Build history of the part. All positions in model axes, mm. Face numbers are marked on the shaded views. A direction names the side the tool comes from. Round coordinates to 2 decimals unless told otherwise and drop trailing zeros. Write each loop counter-clockwise with the first axis right and the second up, starting at its lowest first coordinate (ties: lowest second). Pieces come first, ordered by that corner, then holes. Notation, with made-up numbers: M 47.25,-29 L 71.25,-29 A23 ccw 71.25,2 Z; hole C 51.5,44 d1. An arc over 180 degrees is marked long. One line per item, written item: value. Start each with the question number.
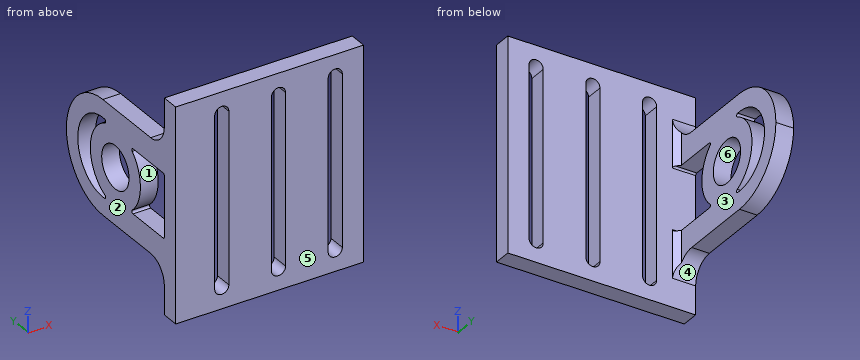
```python
from build123d import *

# Parameters (mm, degrees)
SKETCH1_W           = 48
SKETCH1_H           = 60
BOSS_EXTRUDE1_DEPTH = 5
SKETCH2_W           = 60
SKETCH2_H           = 5
BOSS_EXTRUDE2_DEPTH = 5
SKETCH4_W           = 5
SKETCH4_H           = 32
BOSS_EXTRUDE3_DEPTH = 43
FILLET2_R           = 6
CHAMFER1_SIZE       = 1.5
SKETCH6_R           = 6
CUT_EXTRUDE1_DEPTH  = 94.343451832
FILLET3_R           = 16
CUT_EXTRUDE2_DEPTH  = 94.343451832


with BuildPart() as part:
    # Sketch1 → Boss-Extrude1 (new body)
    with BuildSketch(Plane(origin=(0, 0, 0), x_dir=(1, 0, 0), z_dir=(0, 1, 0))):
        with Locations((24, -30)):
            Rectangle(SKETCH1_W, SKETCH1_H)
        with BuildLine():
            Line((10, -6), (10, -54))
            ThreePointArc((10, -54), (8, -56), (6, -54))
            Line((6, -54), (6, -6))
            ThreePointArc((6, -6), (8, -4), (10, -6))
        make_face(mode=Mode.SUBTRACT)
        with BuildLine():
            Line((38, -6), (38, -54))
            ThreePointArc((38, -54), (40, -56), (42, -54))
            Line((42, -54), (42, -6))
            ThreePointArc((42, -6), (40, -4), (38, -6))
        make_face(mode=Mode.SUBTRACT)
        with BuildLine():
            Line((26, -6), (26, -54))
            ThreePointArc((26, -54), (24, -56), (22, -54))
            Line((22, -54), (22, -6))
            ThreePointArc((22, -6), (24, -4), (26, -6))
        make_face(mode=Mode.SUBTRACT)
    extrude(amount=BOSS_EXTRUDE1_DEPTH)

    # Sketch2 → Boss-Extrude2 (add)
    with BuildSketch(Plane.ZY):
        with Locations((30, 2.5)):
            Rectangle(SKETCH2_W, SKETCH2_H)
    extrude(amount=BOSS_EXTRUDE2_DEPTH)

    # Sketch4 → Boss-Extrude3 (add)
    with BuildSketch(Plane(origin=(0, 5, 0), x_dir=(1, 0, 0), z_dir=(0, 1, 0))):
        with Locations((-2.5, -30)):
            Rectangle(SKETCH4_W, SKETCH4_H)
    extrude(amount=BOSS_EXTRUDE3_DEPTH)

    # Fillet2
    fillet2_edges = [part.edges().sort_by_distance(p)[0] for p in [
        (-2.5, 5, 46),
        (-2.5, 5, 14),
    ]]
    fillet(fillet2_edges, radius=FILLET2_R)

    # Chamfer1
    chamfer1_edges = [part.edges().sort_by_distance(p)[0] for p in [
        (0, 5, 30),
    ]]
    chamfer(chamfer1_edges, length=CHAMFER1_SIZE)

    # Sketch6 → Cut-Extrude1 (cut, through all)
    with BuildSketch(Plane.ZY.offset(5)):
        with Locations((30, 26.5)):
            Circle(SKETCH6_R)
    extrude(amount=-CUT_EXTRUDE1_DEPTH, mode=Mode.SUBTRACT)

    # Fillet3
    fillet3_edges = [part.edges().sort_by_distance(p)[0] for p in [
        (-2.5, 48, 46),
        (-2.5, 48, 14),
    ]]
    fillet(fillet3_edges, radius=FILLET3_R - 0.0001)  # a hair under: the kernel refuses the full size

    # Sketch7 → Cut-Extrude2 (cut, through all)
    with BuildSketch(Plane.ZY.offset(5)):
        with BuildLine():
            Line((21, 18.754033308), (21, 5.5))
            ThreePointArc((21, 5.5), (21.146446609, 5.146446609), (21.5, 5))
            Line((21.5, 5), (38.5, 5))
            ThreePointArc((38.5, 5), (38.853553391, 5.146446609), (39, 5.5))
            Line((39, 5.5), (39, 18.754033308))
            ThreePointArc((39, 18.754033308), (38.68057878, 19.220285712), (38.130434783, 19.090814468))
            ThreePointArc((38.130434783, 19.090814468), (30, 15.5), (21.869565217, 19.090814468))
            ThreePointArc((21.869565217, 19.090814468), (21.31942122, 19.220285712), (21, 18.754033308))
        make_face()
        with BuildLine():
            ThreePointArc((40.971902892, 31.214285714), (30, 43), (19.028097108, 31.214285714))
            ThreePointArc((19.028097108, 31.214285714), (19.438706545, 30.757825209), (19.982175621, 31.043478261))
            ThreePointArc((19.982175621, 31.043478261), (30, 37.5), (40.017824379, 31.043478261))
            ThreePointArc((40.017824379, 31.043478261), (40.561293455, 30.757825209), (40.971902892, 31.214285714))
        make_face()
    extrude(amount=-CUT_EXTRUDE2_DEPTH, mode=Mode.SUBTRACT)


solid = part.part
```
Item 1: Cut at A-A, the plane y = 26.5. Write the cut outline in (x, z).
Item 2: Which spindle directions (+Z, -Z, +X, -X, +Y, -Y) get a long thin tool onto all of the face, cutting with end or side? Do the marked faces 1 and 2. Say none if no direction does.
Item 3: Two-plate mould, pull along Y, no slides. Class the marked faces 3, 4, 5 and 6: pulls with the +Y half, pulls with the -Y half, needs draft (parallel to the pull), parting line crosses it, or undercut.
Item 4: Drop flat-ended pins along their axis: pin 1 (4 mm diameter, centred on x = -2.5, y = 23.5, fed in from +Z); pin 2 (2 mm diameter, centred on y = 32, z = 24.5, fed in from +X); pin 3 (3 mm diameter, centred on x = -0.5, y = 10.5, fed in from -Z); pin 4 (7 mm diameter, centred on y = 26.5, z = 30, fed in from +X). Give the stop position or say it passes through.
Item 5: Cut at D-D, the plane y = 44.5. Write the cut outline in (x, z).
Item 6: Cut at B-B, the plane x = 40. Write the cut outline in (y, z).
Item 7: Drill centre lines: line 1 (Y direction, x = 12, z = 28); line 2 (X direction, y = 39.5, z = 42.5); line 3 (Z direction, x = -1, y = 26). Where is each one in solid material? Low to high.
Item 8: Cut at C-C, the plane x = 31. Write the cut outline in (y, z), plus the area to 3 significant figures.
Computed values:
1. outline: M -5,14 L 0,14 L 0,24 L -5,24 Z; M -5,36 L 0,36 L 0,46 L -5,46 Z
2. face 1: +X, -X
2. face 2: +Z, -Z, -X, +Y, -Y
3. face 3: needs draft
3. face 4: pulls with the +Y half
3. face 5: pulls with the -Y half
3. face 6: undercut
4. pin 1: stops at z = 46
4. pin 2: stops at x = 0
4. pin 3: stops at z = 13.66
4. pin 4: passes through
5. outline: M -5,20.01 L 0,20.01 L 0,39.99 L -5,39.99 Z
6. outline: M 0,0 L 5,0 L 5,4 L 0,4 Z; M 0,56 L 5,56 L 5,60 L 0,60 Z
7. line 1: y = 0 to 5
7. line 2: x = -5 to 0
7. line 3: z = 14 to 24.02, 35.98 to 46
8. outline: M 0,0 L 5,0 L 5,60 L 0,60 Z
8. area: 300 mm2
